Design review of the part built by this model. Coordinates are the model's own, in mm. A direction names the side the tool comes from. Coordinates: 2 decimals unless noted, no trailing zeros. Write each loop counter-clockwise with the first axis right and the second up, starting at its lowest first coordinate (ties: lowest second). Pieces come first, ordered by that corner, then holes.
Q1. Take a section at A-A, the plane x = 103.5. Write out the cut boundary in (y, z).
Q2. Take a section at B-B, the plane z = 5. Write out the cut boundary in (x, y), plus the area to 3 significant figures.
Q3. For L1, parallel to Z at x = 68.5, y = 0.75; L2, parallel to Z at x = 81, y = 0.5; L3, parallel to X at y = 0.5, z = 22.5, list the stretches that pass through material, from the lowest coordinate up.
Q4. Take a section at D-D, the plane x = 77. Write out the cut boundary in (y, z).
Q5. Take a section at C-C, the plane y = 4.25. Write out the cut boundary in (x, z), plus the area to 3 significant figures.
Q6. For faces 4 (the flat face through (65, 6.35, 1)), 5 (the flat face through (95.25, 3, 25)), 6 (the flat face through (38.1, 3, -13)), list the 3-axis set-ups (+Z, -Z, +X, -X, +Y, -Y) from which the entire face can be reached by the end or side of a thin tool; tool diameter is ignored.
Q7. For pin 1 Ø2 at (y, z) = (1.5, 27.5) entering from -X (3 decimals); pin 2 Ø1 at (y, z) = (2.5, 6.5) entering from -X; pin 3 Ø1.9 at (y, z) = (2.5, 26) entering from -X; pin 4 Ø4 at (x, z) = (110, 4) entering from -Y, all flat-tipped, find the tip position at first contact; note any pin that passes through.
Q8. The part is to be moulded in two halves that separate along Z. For faces 1 (the flat face through (57, 3, 50.8)), 2 (the flat face through (69.85, 3, 25)), 3 (the flat face through (111, 3, 0)), say which applies: released by +Z, released by -Z, zero draft, split by the parting line, or undercut.
Autodesk Inventor part; units mm, degrees
sketch "Sketch1" plane through (0, 0, 0) normal (0, 1, 0) x (-1, 0, 0)
  line L0 (0, -50.8) -> (-165.1, -50.8)
  line L1 (-165.1, -50.8) -> (-165.1, 50.8)
  line L2 (-165.1, 50.8) -> (0, 50.8)
  line L3 (0, 50.8) -> (0, -50.8)
  line L4 (0, -71.12) -> (0, 71.12)
  line L5 (-198.12, 0) -> (33.02, 0)
  point P0 (0, 0)
  dimension "d0" = 0
  dimension "d1" = 101.6
  dimension "d2" = 50.8
  dimension "d3" = 165.1
extrude "Extrusion1" add sketch "Sketch1" along normal blind 6.35
chamfer "Chamfer1" distance 76.2 distance2 44.45 1 edges at (0, 3.175, 50.8) measured on face at (0, 2.1167, -16.9333)
chamfer "Chamfer2" distance 44.45 distance2 76.2 1 edges at (165.1, 3.175, 50.8) measured on face at (84.6667, 2.1167, 50.8)
sketch "Sketch2" plane through (0, 6.35, 0) normal (0, 1, 0) x (1, 0, 0)
  line L0 (38.1, 25.4) -> (127, 25.4)
  line L1 (127, 25.4) -> (127, 0)
  line L2 (127, 0) -> (38.1, 0)
  line L3 (38.1, 0) -> (38.1, 25.4)
  line L4 (165.1, 50.8) -> (0, 50.8)
  line L5 (0, 50.8) -> (0, 25.4)
  point P0 (0, 0)
  point P1 (38.1, 12.7)
  dimension "d12" = 25.4
  dimension "d13" = 25.4
  dimension "d14" = 88.9
  dimension "d15" = 38.1
extrude "Extrusion2" cut sketch "Sketch2" against normal up to surface (6.35 mm away)
sketch "Sketch3" plane through (44.45, 0, 50.8) normal (0, 0, 1) x (1, 0, 0)
  line L0 (120.65, 6.35) -> (-44.45, 6.35)
  line L1 (25.4, 6.35) -> (25.4, 0)
  line L2 (25.4, 0) -> (50.8, 0)
  line L3 (50.8, 0) -> (50.8, 6.35)
  line L4 (-44.45, 7.62) -> (-44.45, -1.27)
  point P0 (-44.45, 0)
  dimension "d18" = 25.4
  dimension "d19" = 69.85
sketch "Sketch4" plane through (127, 6.35, 0) normal (0, 0, -1) x (-1, 0, 0)
  line L0 (88.9, -6.35) -> (0, -6.35)
  line L1 (88.9, 0) -> (88.9, -6.35)
  line L2 (0, 0) -> (88.9, 0)
  line L3 (0, 0) -> (0, -6.35)
  line L4 (31.75, -6.35) -> (31.75, 0)
  line L5 (57.15, 0) -> (57.15, -6.35)
  point P0 (127, -6.35)
extrude "Extrusion3" cut sketch "Sketch4" against normal up to next contours L0 L4 L2 L5
equation "\"d2\" = 0.5 * d1"
properties part number "chap3ex1"
Responses:
1. outline: (0, -50.8) - (6.35, -50.8) - (6.35, -25.4) - (0, -25.4) - close; (0, 0) - (6.35, 0) - (6.35, 50.8) - (0, 50.8) - close
2. outline: (17.73, 0) - (69.85, 0) - (69.85, 6.35) - (17.73, 6.35) - close; (95.25, 0) - (147.37, 0) - (147.37, 6.35) - (95.25, 6.35) - close
2. area: 662 mm2
3. L1: z = -50.8 to -25.4, 0 to 50.8
3. L2: z = -50.8 to -25.4
3. L3: x = 27.94 to 69.85, 95.25 to 137.16
4. outline: (0, -50.8) - (6.35, -50.8) - (6.35, -25.4) - (0, -25.4) - close
5. outline: (0, -50.8) - (165.1, -50.8) - (165.1, -25.4) - (120.65, 50.8) - (95.25, 50.8) - (95.25, 0) - (127, 0) - (127, -25.4) - (38.1, -25.4) - (38.1, 0) - (69.85, 0) - (69.85, 50.8) - (44.45, 50.8) - (0, -25.4) - close
5. area: 9,840 mm2
6. face 4: +Z, -Z, +X, -X, +Y
6. face 5: +Z, +Y, -Y
6. face 6: +Y, -Y
7. pin 1: stops at x = 30.275
7. pin 2: stops at x = 18.32
7. pin 3: stops at x = 29.43
7. pin 4: stops at y = 0
8. face 1: released by +Z
8. face 2: zero draft
8. face 3: undercut
